from build123d import *

# Parameters (mm, degrees)
SKETCH1_R           = 3.175
BOSS_EXTRUDE1_DEPTH = 5.953125
THREAD1_PITCH       = 1.27


with BuildPart() as part:
    # Sketch1 → Boss-Extrude1 (new body)
    with BuildSketch(Plane(origin=(0, 0, 0), x_dir=(1, 0, 0), z_dir=(0, 1, 0))):
        Polygon((0, 6.415804866), (-5.55625, 3.207902433), (-5.55625, -3.207902433), (0, -6.415804866), (5.55625, -3.207902433), (5.55625, 3.207902433), align=None)
        with Locations(Location((0, 0, 0), (0, 0, 270))):
            Circle(SKETCH1_R, mode=Mode.SUBTRACT)
    extrude(amount=BOSS_EXTRUDE1_DEPTH)

    # Thread1: the profile of Thread Profile1 profile screwed along a right-hand helix of 4.6875 turns, 8 arcs to a turn; built about Z, then put on its axis
    thread1_z = Axis((0, 0, 0), (0, 0, 1))
    thread1_corners = [(3.1753, 0, -0.000173205), (3.1753, 0, 1.111423202), (2.487592339, 0, 0.714374998), (2.487592339, 0, 0.396874998)]
    with BuildLine(mode=Mode.PRIVATE) as thread1_profile:
        Line(thread1_corners[0], thread1_corners[1])
        Line(thread1_corners[1], thread1_corners[2])
        Line(thread1_corners[2], thread1_corners[3])
        Line(thread1_corners[3], thread1_corners[0])
    thread1_cap = Face(thread1_profile.wire())
    thread1_turn_angles = [0, 22.5, 45, 67.5, 90, 112.5, 135, 157.5, 180, 202.5, 225, 247.5, 270, 292.5, 315, 337.5, 360]
    thread1_turn_weights = [1, 0.9238795325112867, 1, 0.9238795325112867, 1, 0.9238795325112867, 1, 0.9238795325112867, 1, 0.9238795325112867, 1, 0.9238795325112867, 1, 0.9238795325112867, 1, 0.9238795325112867, 1]
    thread1_turn_rails = [Edge.make_bspline([Vector(p[0], p[1], 0).rotate(thread1_z, thread1_turn_angles[k]) / thread1_turn_weights[k] + Vector(0, 0, p[2] + THREAD1_PITCH * thread1_turn_angles[k] / 360) for k in range(17)], [0, 0, 0, 1, 1, 2, 2, 3, 3, 4, 4, 5, 5, 6, 6, 7, 7, 8, 8, 8], 2, thread1_turn_weights) for p in thread1_corners]
    thread1_turn_sides = [Face.make_surface_from_curves(thread1_turn_rails[p[0]], thread1_turn_rails[p[1]]) for p in [(0, 1), (1, 2), (2, 3), (3, 0)]]
    thread1_last_angles = [1440, 1462.5, 1485, 1507.5, 1530, 1552.5, 1575, 1597.5, 1620, 1642.5, 1665, 1676.25, 1687.5]
    thread1_last_weights = [1, 0.9238795325112867, 1, 0.9238795325112867, 1, 0.9238795325112867, 1, 0.9238795325112867, 1, 0.9238795325112867, 1, 0.9807852804032304, 1]
    thread1_last_rails = [Edge.make_bspline([Vector(p[0], p[1], 0).rotate(thread1_z, thread1_last_angles[k]) / thread1_last_weights[k] + Vector(0, 0, p[2] + THREAD1_PITCH * thread1_last_angles[k] / 360) for k in range(13)], [0, 0, 0, 1, 1, 2, 2, 3, 3, 4, 4, 5, 5, 6, 6, 6], 2, thread1_last_weights) for p in thread1_corners]
    thread1_last_sides = [Face.make_surface_from_curves(thread1_last_rails[p[0]], thread1_last_rails[p[1]]) for p in [(0, 1), (1, 2), (2, 3), (3, 0)]]
    thread1 = Plane(origin=(0, 5.953125, 0), x_dir=(-1, 0, 0), z_dir=(0, -1, 0)) * Solid(Shell([*[p.moved(Location((0, 0, THREAD1_PITCH * i))) for i in range(4) for p in thread1_turn_sides], *thread1_last_sides, thread1_cap, thread1_cap.rotate(thread1_z, 1687.5).moved(Location((0, 0, THREAD1_PITCH * 1687.5 / 360)))]))
    add(thread1)


solid = part.part
The model under review builds one solid part; all positions refer to its coordinate system, in mm. Round coordinates to 2 decimals unless told otherwise and drop trailing zeros. Loops run counter-clockwise (first coordinate to the right, second up) from the corner with the lowest first, then second, coordinate; pieces in that order, holes last. Notation, with made-up numbers: (-27, 39) -> (-8, 39) arc R21 ccw to (-8, 71) -> close; hole circle Ø2 at (55, 34.25). An arc over 180 degrees is marked (long way). One line per question, with ' | ' between items. Start each with the question number.
Item 1: Wall thickness on line 1 along Y through (x, z) = (3, 2); line 2 along X through (y, z) = (3, 1.5); line 3 along Z through (x, y) = (1, 3): over which ranges is each line inside the solid? List them lowest first. Write a range as [from, to].
Item 2: Add section B-B, the plane z = 5.75. Write out the cut boundary in (x, y).
Item 3: Add section A-A, the plane x = 4.25. Write out the cut boundary in (y, z).
Item 4: Add section C-C, the plane x = -3. Count the separate pieces of the cut face and the enclosed holes in it, then the cut area to 3 significant figures.
Item 5: For pin 1 (2 mm diameter, centred on x = 3.5, y = 4.5, fed in from +Z); pin 2 (3 mm diameter, centred on x = -0.5, z = -1, fed in from -Y), all flat-tipped, find the tip position at first contact; note any pin that passes through.
Return value:
1) line 1: y = [0, 5.95] | line 2: x = [-5.56, -1.98], [2.45, 5.56] | line 3: z = [-5.84, -2.96], [2.46, 5.84]
2) outline: (-1.15, 0) -> (1.15, 0) -> (1.15, 5.95) -> (-1.15, 5.95) -> close
3) outline: (0, -3.96) -> (5.95, -3.96) -> (5.95, 3.96) -> (0, 3.96) -> close
4) separate pieces: 1 | enclosed holes: 3 | area: 52.5 mm2
5) pin 1: stops at z = 4.97 | pin 2: stops at y = -0.16
